Build history of the part. All positions in model axes, mm. A direction names the side the tool comes from. Give positions to 0.01 mm unless a question says otherwise; leave off trailing zeros. Loops run counter-clockwise (first coordinate to the right, second up) from the corner with the lowest first, then second, coordinate; pieces in that order, holes last. Notation, with made-up numbers: (8.5, 26) -> (60.5, 26) arc R16 ccw to (60.5, 32) -> close; hole circle Ø10 at (-29.5, 10). An arc over 180 degrees is marked (long way). Answer as a JSON object with one key per item and string values. Group by question number.
Q1. Band-saw the part on A-A, the plane x = 1. Write the cut outline in (y, z) (3 decimals), plus the area to 3 significant figures.
Q2. Wall check: probe 1 along X at (y, z) = (7, 50); probe 2 along Y at (x, z) = (8, 20) (3 decimals). Give the ranges that are in metal, low to high. Write a range as from..to.
Q3. Band-saw the part on C-C, the plane y = 15. Write the cut outline in (x, z).
Q4. Band-saw the part on B-B, the plane z = 17. Write the cut outline in (x, y) (3 decimals), plus the area to 3 significant figures.
Q5. Band-saw the part on D-D, the plane x = 11. Write the cut outline in (y, z) (3 decimals), plus the area to 3 significant figures.
Q6. Drop flat-ended pins along their axis: pin 1 (3.5 mm diameter, centred on x = -17.5, z = 18, fed in from -Y) (3 decimals); pin 2 (3 mm diameter, centred on x = 4.5, z = 25.5, fed in from +Y) (3 decimals); pin 3 (1.1 mm diameter, centred on x = -13, z = 18.5, fed in from -Y); pin 4 (6.5 mm diameter, centred on y = 17, z = 24.5, fed in from -X). Give the stop position or say it passes through.
Q7. Tool access for faces 1 (the flat face through (0, 19.975, 20)), 2 (the flat face through (-1, 13.975, 17)), 3 (the flat face through (7, 17, 26.5)): list every direction of +Z, -Z, +X, -X, +Y, -Y with a clear straight run to the whole face (end or side of a thin tool).
Q8. Two-plate mould, pull along Y, no slides. Class faces 4 (the cylindrical face through (-19.2, 17, 17)), 5 (the flat face through (10, 4, 36)), 6 (the flat face through (-4, 10.85, 17)): pulls with the +Y half, pulls with the -Y half, needs draft (parallel to the pull), parting line crosses it, or undercut.
from build123d import *

# Parameters (mm, degrees)
BOSS_EXTRUDE1_START     = 13.5
BOSS_EXTRUDE1_DEPTH     = 7
BOSS_EXTRUDE2_START     = 20.5
SKETCH2_W               = 8
SKETCH2_H               = 6
BOSS_EXTRUDE2_DEPTH     = 6
BOSS_EXTRUDE3_START     = 21.5
SKETCH3_W               = 3
SKETCH3_H               = 31.975
BOSS_EXTRUDE3_DEPTH     = 30
CUT_EXTRUDE1_DEPTH      = 60.835195537
CUT_EXTRUDE1_DEPTH_BACK = 60.835195537
SKETCH4_W               = 20
SKETCH4_H               = 2.4
CUT_EXTRUDE2_DEPTH      = 60.835195537
CUT_EXTRUDE2_DEPTH_BACK = 60.835195537
SKETCH5_R               = 1.2


with BuildPart() as part:
    # Sketch1 → Boss-Extrude1 (new body)
    with BuildSketch(Plane.XY.offset(BOSS_EXTRUDE1_START)):
        Polygon((-23, 19.975), (13, 19.975), (13, 13.975), (7.70102766, 13.975), (6.563620678, 10.85), (5.217351773, 10.85), (4.079944791, 13.975), (2.988638679, 13.975), (1.851231697, 10.85), (0.504962793, 10.85), (-0.632444189, 13.975), (-1.723750301, 13.975), (-2.861157283, 10.85), (-4.207426188, 10.85), (-5.34483317, 13.975), (-6.436139281, 13.975), (-7.573546263, 10.85), (-8.919815168, 10.85), (-10.05722215, 13.975), (-11.148528262, 13.975), (-12.285935244, 10.85), (-13.632204148, 10.85), (-14.76961113, 13.975), (-23, 13.975), align=None)
    extrude(amount=BOSS_EXTRUDE1_DEPTH)

    # Sketch2 → Boss-Extrude2 (add)
    with BuildSketch(Plane.XY.offset(BOSS_EXTRUDE2_START)):
        with Locations((9, 16.975)):
            Rectangle(SKETCH2_W, SKETCH2_H)
    extrude(amount=BOSS_EXTRUDE2_DEPTH)

    # Sketch3 → Boss-Extrude3 (add)
    with BuildSketch(Plane.XY.offset(BOSS_EXTRUDE3_START)):
        with Locations((11.5, 3.9875)):
            Rectangle(SKETCH3_W, SKETCH3_H)
    extrude(amount=BOSS_EXTRUDE3_DEPTH)

    # Sketch4 → Cut-Extrude1 (cut, two sides: drawn at the far end of the back side and taken through both)
    with BuildSketch(Plane.XY.offset(-CUT_EXTRUDE1_DEPTH_BACK)):
        with Locations((-8, 16.975)):
            Rectangle(SKETCH4_W, SKETCH4_H)
    extrude(amount=CUT_EXTRUDE1_DEPTH + CUT_EXTRUDE1_DEPTH_BACK, mode=Mode.SUBTRACT)

    # Sketch5 → Cut-Extrude2 (cut, two sides: drawn at the far end of the back side and taken through both)
    with BuildSketch(Plane.XY.offset(-CUT_EXTRUDE2_DEPTH_BACK)):
        with Locations((-18, 16.975)):
            Circle(SKETCH5_R)
        with Locations((2, 16.975)):
            Circle(SKETCH5_R)
    extrude(amount=CUT_EXTRUDE2_DEPTH + CUT_EXTRUDE2_DEPTH_BACK, mode=Mode.SUBTRACT)


solid = part.part
Worked answers:
{
 "1": {"outline": "(10.85, 13.5) -> (15.775, 13.5) -> (15.775, 20.5) -> (10.85, 20.5) -> close; (18.175, 13.5) -> (19.975, 13.5) -> (19.975, 20.5) -> (18.175, 20.5) -> close", "area": "47.1 mm2"},
 "2": {"probe 1": "10..13", "probe 2": "13.975..19.975"},
 "3": {"outline": "(-23, 13.5) -> (13, 13.5) -> (13, 51.5) -> (10, 51.5) -> (10, 26.5) -> (5, 26.5) -> (5, 20.5) -> (-23, 20.5) -> close"},
 "4": {"outline": "(-23, 13.975) -> (-14.77, 13.975) -> (-13.632, 10.85) -> (-12.286, 10.85) -> (-11.149, 13.975) -> (-10.057, 13.975) -> (-8.92, 10.85) -> (-7.574, 10.85) -> (-6.436, 13.975) -> (-5.345, 13.975) -> (-4.207, 10.85) -> (-2.861, 10.85) -> (-1.724, 13.975) -> (-0.632, 13.975) -> (0.505, 10.85) -> (1.851, 10.85) -> (2.989, 13.975) -> (4.08, 13.975) -> (5.217, 10.85) -> (6.564, 10.85) -> (7.701, 13.975) -> (13, 13.975) -> (13, 19.975) -> (-23, 19.975) -> close; hole (-18, 15.775) -> (2, 15.775) arc R1.2 ccw to (2, 18.175) -> (-18, 18.175) arc R1.2 ccw to start", "area": "202 mm2"},
 "5": {"outline": "(-12, 21.5) -> (13.975, 21.5) -> (13.975, 13.5) -> (19.975, 13.5) -> (19.975, 51.5) -> (-12, 51.5) -> close", "area": "1,010 mm2"},
 "6": {"pin 1": "y = 13.975", "pin 2": "y = 19.975", "pin 3": "y = 10.85", "pin 4": "x = 5"},
 "7": {"face 1": "+Z, -Z, +X, -X, +Y", "face 2": "+Z, -Z, -Y", "face 3": "+Z, -X, +Y, -Y"},
 "8": {"face 4": "undercut", "face 5": "needs draft", "face 6": "pulls with the -Y half"}
}
